Can you work these out from the model? Positions are in its coordinate system, mm. Face numbers are marked on the shaded views. Round coordinates to 2 decimals unless told otherwise and drop trailing zeros. Order: outer loops, then holes, each group sorted by start corner. A loop starts at its lowest first (then second) coordinate and runs counter-clockwise, first axis right, second up. Notation, with made-up numbers: M 2,-0.5 L 22,-0.5 A28 cw 22,28.5 Z; hole C 86,27.25 d5. An arc over 180 degrees is marked long. One line per question, with ' | ' between items.
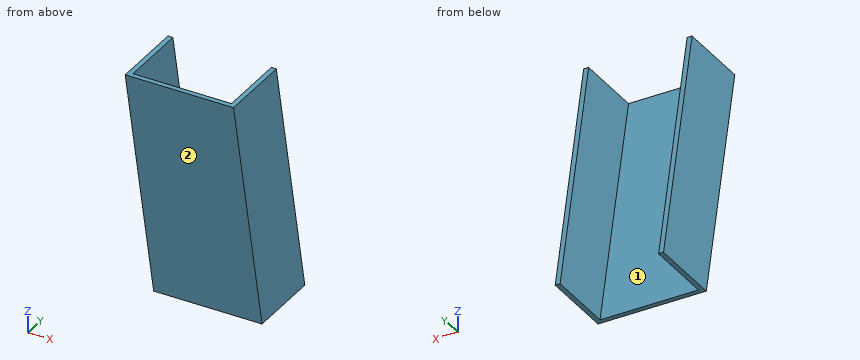
```python
from build123d import *


with BuildPart() as part:
    # Sketch2 → Loft3 section 0
    with BuildSketch(Plane.XY.offset(100)):
        with BuildLine():
            Line((44, 10), (44, -20))
            Line((44, -20), (0, -20))
            Line((0, -20), (0, 10))
            Line((0, 10), (2, 10))
            Line((2, 10), (2, -18))
            Line((2, -18), (42, -18))
            Line((42, -18), (42, 10))
            Line((42, 10), (44, 10))
        make_face()
    # Sketch1 → Loft3 section 1
    with BuildSketch(Plane.XY):
        with BuildLine():
            Line((44, 30), (44, 0))
            Line((44, 0), (0, 0))
            Line((0, 0), (0, 30))
            Line((0, 30), (2, 30))
            Line((2, 30), (2, 2))
            Line((2, 2), (42, 2))
            Line((42, 2), (42, 30))
            Line((42, 30), (44, 30))
        make_face()
    loft()


solid = part.part
```
(1) If we section it at A-A on x = 13: Please give me the cut outline in (y, z).
Final values:
outline: M -20,100 L 0,0 L 2,0 L -18,100 Z
(2) Please list where these lines run through material, in increasing order: probe 1 along X at (y, z) = (16, 62); probe 2 along Y at (x, z) = (19, 46.5); probe 3 along Y at (x, z) = (40.5, 79.5). Write a range as [from, to].
Final values:
probe 1: [0, 2], [42, 44] | probe 2: [-9.3, -7.3] | probe 3: [-15.9, -13.9]
(3) Will these pins go through, and if not, where does the flat tip stop? pin 1 Ø5 at (y, z) = (-4.5, 72) entering from -X; pin 2 Ø8 at (y, z) = (-13.5, 33) entering from -X; pin 3 Ø6 at (x, z) = (36.5, 45.5) entering from -Y; pin 4 Ø12 at (x, z) = (20.5, 19.5) entering from -Y.
Final values:
pin 1: x = 0 | pin 2: through | pin 3: y = -9.7 | pin 4: y = -5.1
(4) Thinking about a two-plate mould opening in X: for the marked faces 1 and 2, which applies, released by +X, released by -X, zero draft, split by the parting line, or undercut?
Final values:
face 1: undercut | face 2: zero draft
